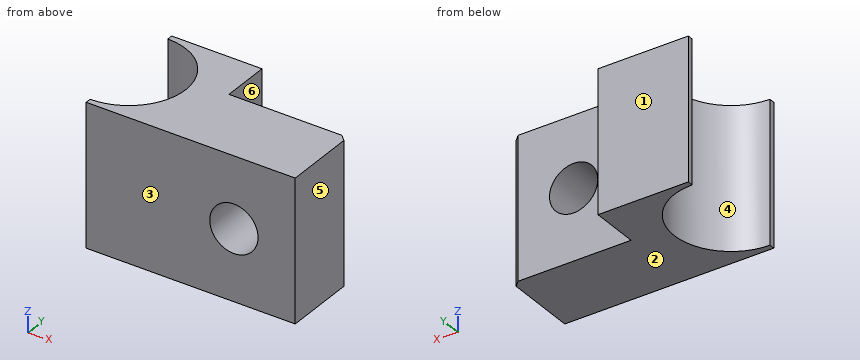
```python
from build123d import *

# Parameters (mm, degrees)
BOSS_EXTRUDE1_DEPTH      = 31.75
X_0_397_DIAMETER_HOLE1_D = 10.795
CHAMFER1_SIZE            = 1.27


with BuildPart() as part:
    # Sketch1 → Boss-Extrude1 (new body)
    with BuildSketch(Plane.XY):
        with BuildLine():
            Line((46.736, 0), (46.736, 17.145))
            Line((46.736, 17.145), (20.193, 17.145))
            Line((20.193, 17.145), (20.193, 27.94))
            Line((20.193, 27.94), (0, 27.94))
            Line((0, 27.94), (0, 26.67))
            ThreePointArc((0, 26.67), (12.7, 13.97), (0, 1.27))
            Line((0, 1.27), (0, 0))
            Line((0, 0), (46.736, 0))
        make_face()
    extrude(amount=BOSS_EXTRUDE1_DEPTH)

    # X (0.397) Diameter Hole1 (through all)
    with Locations(Plane(origin=(0, 17.145, 0), x_dir=(1, 0, 0), z_dir=(0, 1, 0))):
        with Locations((33.02, -15.875)):
            Hole(X_0_397_DIAMETER_HOLE1_D / 2)

    # Chamfer1
    chamfer1_edges = [part.edges().sort_by_distance(p)[0] for p in [
        (46.736, 17.145, 15.875),
    ]]
    chamfer(chamfer1_edges, length=CHAMFER1_SIZE)


solid = part.part
```
Could you check a few things on this model? Use its own coordinates, in mm. Face numbers are marked on the shaded views. A direction names the side the tool comes from. Give positions to 0.01 mm unless a question says otherwise; leave off trailing zeros. Write each loop counter-clockwise with the first axis right and the second up, starting at its lowest first coordinate (ties: lowest second). Pieces come first, ordered by that corner, then holes. Notation, with made-up numbers: (-29, 77.5) - (16, 77.5) arc R35 ccw to (16, 112.5) - close; hole circle Ø1 at (-30.5, -13). An arc over 180 degrees is marked (long way). One line per item, written item: value. Start each with the question number.
Item 1: If we mould it in two halves opening along Y, with no side actions, what happens to the marked faces 1, 2, 3 and 4? For each: +Y half, -Y half, draft (parallel to the pull), parting line (faces both ways), or undercut.
Item 2: I'm going to push flat-ended pins straight in: pin 1 (4 mm diameter, centred on x = 30.5, y = 19.5, fed in from +Z); pin 2 (8.5 mm diameter, centred on y = 22, z = 16, fed in from +X). Where does each tip first touch, or does it pass through?
Item 3: Which directions (+Z, -Z, +X, -X, +Y, -Y) give clear straight access to the entire face, cutting with the end or side of a thin tool? Please do the marked faces 5 and 6.
Item 4: Imagine slicing it at B-B, the plane z = 18.5. List the corners of the cut face in (x, y) for me (3 decimals).
Item 5: Please list where these lines run through material, in increasing order: line 1 (Z direction, x = 33.02, y = 7.5); line 2 (Y direction, x = 5, z = 26); line 3 (Y direction, x = 27, z = 12.5) (3 decimals). Write a range as from..to.
Item 6: Imagine slicing it at D-D, the plane z = 29. List the corners of the cut face in (x, y) for me (3 decimals).
Geometry says:
1. face 1: +Y half
1. face 2: draft
1. face 3: -Y half
1. face 4: undercut
2. pin 1: through
2. pin 2: x = 20.19
3. face 5: +Z, -Z, +X, +Y, -Y
3. face 6: +Z, -Z, +X, +Y
4. outline: (0, 0) - (28.304, 0) - (28.304, 17.145) - (20.193, 17.145) - (20.193, 27.94) - (0, 27.94) - (0, 26.67) arc R12.7 cw to (0, 1.27) - close; (37.736, 0) - (46.736, 0) - (46.736, 15.875) - (45.466, 17.145) - (37.736, 17.145) - close
5. line 1: 0..10.48, 21.27..31.75
5. line 2: 0..2.3, 25.64..27.94
5. line 3: 0..17.145
6. outline: (0, 0) - (46.736, 0) - (46.736, 15.875) - (45.466, 17.145) - (20.193, 17.145) - (20.193, 27.94) - (0, 27.94) - (0, 26.67) arc R12.7 cw to (0, 1.27) - close
